```python
from build123d import *

# Parameters (mm, degrees)
SKETCH1_R           = 3.2
BOSS_EXTRUDE1_DEPTH = 3
CUT_EXTRUDE1_DEPTH  = 2
FILLET1_R           = 6
FILLET2_R           = 1
FILLET3_R           = 0.5


with BuildPart() as part:
    # Sketch1 → Boss-Extrude1 (new body)
    with BuildSketch(Plane(origin=(0, 0, 0), x_dir=(1, 0, 0), z_dir=(0, 1, 0))):
        with BuildLine():
            Line((-17.5, -17.5), (17.5, -17.5))
            Line((17.5, -17.5), (29.489041807, -3.981017917))
            ThreePointArc((29.489041807, -3.981017917), (31, 0), (29.489041807, 3.981017917))
            Line((29.489041807, 3.981017917), (17.5, 17.5))
            Line((17.5, 17.5), (-17.5, 17.5))
            Line((-17.5, 17.5), (-29.489041807, 3.981017917))
            ThreePointArc((-29.489041807, 3.981017917), (-31, 0), (-29.489041807, -3.981017917))
            Line((-29.489041807, -3.981017917), (-17.5, -17.5))
        make_face()
        with Locations((-25, 0)):
            Circle(SKETCH1_R, mode=Mode.SUBTRACT)
        with Locations((25, 0)):
            Circle(SKETCH1_R, mode=Mode.SUBTRACT)
    extrude(amount=BOSS_EXTRUDE1_DEPTH)

    # Sketch2 → Cut-Extrude1 (cut)
    with BuildSketch(Plane(origin=(0, 3, 0), x_dir=(1, 0, 0), z_dir=(0, 1, 0))):
        Polygon((-15.2, 15.2), (-7.7, 15.2), (-7.7, 17.5), (7.7, 17.5), (7.7, 15.2), (15.2, 15.2), (15.2, -15.2), (-15.2, -15.2), align=None)
    extrude(amount=-CUT_EXTRUDE1_DEPTH, mode=Mode.SUBTRACT)

    # Fillet1
    fillet1_edges = [part.edges().sort_by_distance(p)[0] for p in [
        (17.5, 1.5, 17.5),
        (-17.5, 1.5, 17.5),
        (-17.5, 1.5, -17.5),
        (17.5, 1.5, -17.5),
    ]]
    fillet(fillet1_edges, radius=FILLET1_R)

    # Fillet2
    fillet2_edges = [part.edges().sort_by_distance(p)[0] for p in [
        (-7.7, 2, -15.2),
        (7.7, 2, -15.2),
    ]]
    fillet(fillet2_edges, radius=FILLET2_R)

    # Fillet3
    fillet3_edges = [part.edges().sort_by_distance(p)[0] for p in [
        (-11.95, 3, -15.2),
        (-7.992893219, 3, -15.492893219),
        (7.992893219, 3, -15.492893219),
        (15.2, 3, 0),
        (11.95, 3, -15.2),
        (-7.7, 3, -16.85),
        (-15.2, 3, 0),
        (0, 3, 15.2),
        (7.7, 3, -16.85),
    ]]
    fillet(fillet3_edges, radius=FILLET3_R)


solid = part.part
```
Here's how the part is built. I have some questions about the finished solid (model axes, mm). A direction names the side the tool comes from. Round coordinates to 2 decimals unless told otherwise and drop trailing zeros. Write each loop counter-clockwise with the first axis right and the second up, starting at its lowest first coordinate (ties: lowest second). Pieces come first, ordered by that corner, then holes.
Q1. Will these pins go through, and if not, where does the flat tip stop? P1, Ø1.2, axis at y = 1.5, z = 4, coming from the +X side; P2, Ø1.5, axis at x = -0.5, z = -2, coming from the +Y side; P3, Ø1.6, axis at x = -3.5, y = 2, coming from the -Z side; P4, Ø10, axis at x = -25, z = 0, coming from the -Y side.
Q2. If we section it at A-A on y = 1.75: Write out the boundary of the cut face in (x, z).
Q3. Please list where these lines run through material, in increasing order: probe 1 along X at (y, z) = (0.9, 0); probe 2 along X at (y, z) = (2.4, 0); probe 3 along Z at (x, y) = (15, 0.3).
Q4. If we section it at B-B on z = 0: Write out the boundary of the cut face in (x, y), plus the area to 3 significant figures.
Q5. If we mould it in two halves opening along X, with no side actions, what happens to faces 1 (the flat face through (24.46, 1.48, -9.65)), 2 (the flat face through (15.2, 2, 0)), 3 (the flat face through (-24.32, 1.48, -9.81))? For each: +X half, -X half, draft (parallel to the pull), parting line (faces both ways), or undercut.
Q6. Which directions (+Z, -Z, +X, -X, +Y, -Y) give clear straight access to the entire face, cutting with the end or side of a thin tool? Please do faces 4 (the flat face through (-12, 2, -15.2)), 5 (the cylindrical face through (-28.2, 1.5, -0.1)), 6 (the flat face through (7.7, 2, -17)).
Q7. If we section it at C-C on x = -27: Write out the boundary of the cut face in (y, z).
Q8. If we section it at D-D on x = -7: Write out the boundary of the cut face in (y, z).
Answer below:
1. P1: stops at x = 29.94
1. P2: stops at y = 1
1. P3: stops at z = 15.2
1. P4: stops at y = 0
2. outline: (-29.49, -3.98) - (-19.29, -15.48) arc R6 ccw to (-14.8, -17.5) - (-7.7, -17.5) - (-7.7, -16.2) arc R1 ccw to (-8.7, -15.2) - (-15.2, -15.2) - (-15.2, 15.2) - (15.2, 15.2) - (15.2, -15.2) - (8.7, -15.2) arc R1 ccw to (7.7, -16.2) - (7.7, -17.5) - (14.8, -17.5) arc R6 ccw to (19.29, -15.48) - (29.49, -3.98) arc R6 ccw to (29.49, 3.98) - (19.29, 15.48) arc R6 ccw to (14.8, 17.5) - (-14.8, 17.5) arc R6 ccw to (-19.29, 15.48) - (-29.49, 3.98) arc R6 ccw to start; hole circle Ø6.4 at (-25, 0); hole circle Ø6.4 at (25, 0)
3. probe 1: x = -31 to -28.2, -21.8 to 21.8, 28.2 to 31
3. probe 2: x = -31 to -28.2, -21.8 to -15.2, 15.2 to 21.8, 28.2 to 31
3. probe 3: z = -17.5 to 17.5
4. outline: (-31, 0) - (-28.2, 0) - (-28.2, 3) - (-31, 3) - close; (-21.8, 0) - (21.8, 0) - (21.8, 3) - (15.7, 3) arc R0.5 ccw to (15.2, 2.5) - (15.2, 1) - (-15.2, 1) - (-15.2, 2.5) arc R0.5 ccw to (-15.7, 3) - (-21.8, 3) - close; (28.2, 0) - (31, 0) - (31, 3) - (28.2, 3) - close
4. area: 86.7 mm2
5. face 1: +X half
5. face 2: undercut
5. face 3: -X half
6. face 4: +Y
6. face 5: +Y, -Y
6. face 6: -Z, +Y
7. outline: (0, -6.79) - (3, -6.79) - (3, -2.5) - (0, -2.5) - close; (0, 2.5) - (3, 2.5) - (3, 6.79) - (0, 6.79) - close
8. outline: (0, -17.5) - (1, -17.5) - (1, 15.2) - (2.5, 15.2) arc R0.5 ccw to (3, 15.7) - (3, 17.5) - (0, 17.5) - close
